```python
from build123d import *

# Parameters (mm, degrees)
SKETCH1_W                = 23.7998
SKETCH1_H                = 9.525
BOSS_EXTRUDE1_DEPTH      = 4.7625
BOSS_EXTRUDE1_DEPTH_BACK = 4.7625
SKETCH2_W                = 14.2748
SKETCH2_H                = 5.08
CUT_EXTRUDE1_DEPTH       = 4.7625
CUT_EXTRUDE1_DEPTH_BACK  = 4.7625
HOLE1_D                  = 3.96748
HOLE1_DEPTH              = 7.874
HOLE1_CSINK_D            = 4.826
HOLE1_CSINK_ANGLE        = 90
HOLE2_D                  = 3.96748
HOLE2_DEPTH              = 1.651
HOLE3_D                  = 4.826
HOLE3_DEPTH              = 9.525


with BuildPart() as part:
    # Sketch1 → Boss-Extrude1 (new body, two sides)
    with BuildSketch(Plane.XY) as boss_extrude1_sk:
        with Locations((7.1501, 0)):
            Rectangle(SKETCH1_W, SKETCH1_H)
    extrude(amount=BOSS_EXTRUDE1_DEPTH)
    extrude(boss_extrude1_sk.sketch, amount=-BOSS_EXTRUDE1_DEPTH_BACK)

    # Sketch2 → Cut-Extrude1 (cut, two sides)
    with BuildSketch(Plane(origin=(0, 0, 0), x_dir=(1, 0, 0), z_dir=(0, 1, 0))) as cut_extrude1_sk:
        with Locations((2.3876, 0)):
            Rectangle(SKETCH2_W, SKETCH2_H)
    extrude(amount=CUT_EXTRUDE1_DEPTH, mode=Mode.SUBTRACT)
    extrude(cut_extrude1_sk.sketch, amount=-CUT_EXTRUDE1_DEPTH_BACK, mode=Mode.SUBTRACT)

    # Hole1
    with Locations(Plane(origin=(19.05, 0, 0), x_dir=(0, 0, -1), z_dir=(1, 0, 0))):
        with Locations((0, 0)):
            CounterSinkHole(HOLE1_D / 2, HOLE1_CSINK_D / 2, depth=HOLE1_DEPTH, counter_sink_angle=HOLE1_CSINK_ANGLE)

    # Hole2
    with Locations(Plane(origin=(11.176, 0, 0), x_dir=(0, 0, -1), z_dir=(1, 0, 0))):
        with Locations((0, 0)):
            Hole(HOLE2_D / 2, depth=HOLE2_DEPTH)

    # Hole3
    with Locations(Plane(origin=(0, 0, -4.7625), x_dir=(-1, 0, 0), z_dir=(0, 0, -1))):
        with Locations((0, 0)):
            Hole(HOLE3_D / 2, depth=HOLE3_DEPTH)

    # Sketch9 → Cut-Revolve1 (revolve, cut)
    with BuildSketch(Plane.XY):
        with BuildLine():
            Line((19.05, 0), (19.05, 4.7625))
            ThreePointArc((19.05, 4.7625), (18.092047749, 7.310175466), (16.51, 9.525))
            Line((16.51, 9.525), (23.8125, 9.525))
            Line((23.8125, 9.525), (23.8125, 0))
            Line((23.8125, 0), (19.05, 0))
        make_face()
    revolve(axis=Axis((23.8125, 0, 0), (-1, 0, 0)), mode=Mode.SUBTRACT)

    # Sketch10 → Cut-Revolve2 (revolve, cut)
    with BuildSketch(Plane.XY):
        with BuildLine():
            Line((-9.5123, 0), (-9.5123, 9.525))
            Line((-9.5123, 9.525), (-2.2098, 9.525))
            ThreePointArc((-2.2098, 9.525), (-3.791847749, 7.310175466), (-4.7498, 4.7625))
            Line((-4.7498, 4.7625), (-4.7498, 0))
            Line((-4.7498, 0), (-9.5123, 0))
        make_face()
    revolve(axis=Axis((-4.7498, 0, 0), (-1, 0, 0)), mode=Mode.SUBTRACT)


solid = part.part
```
Geometry: final body of the model. Coordinates: model frame, mm. A direction names the side the tool comes from. Coordinates: 2 decimals unless noted, no trailing zeros. Order: outer loops, then holes, each group sorted by start corner. A loop starts at its lowest first (then second) coordinate and runs counter-clockwise, first axis right, second up. Notation, with made-up numbers: (84, 57.25) - (124, 57.25) arc R13 ccw to (124, 70.25) - close; hole circle Ø3 at (-25.5, -0.5). An arc over 180 degrees is marked (long way). Return JSON: item names as keys, results as strings. Group by question number.
1. Pull-direction query (Y, two-part tool) for faces 3 (the face through (-1.915, -1.468, 3.667)), 4 (the face through (10, -4.762, 0)), 5 (the face through (4, 0, 2.54)); classes: pulls with the +Y half, pulls with the -Y half, needs draft (parallel to the pull), parting line crosses it, or undercut.
2. Pin query (flat end, axial travel): pin 1 (4.5 mm diameter, centred on y = 0, z = 0, fed in from -X) (3 decimals); pin 2 (4.5 mm diameter, centred on x = 0, y = 0, fed in from -Z). Return the tip coordinate at first contact, or that it passes through.
3. Set-up query: faces 1 (the face through (-4.75, 0, 3)), 2 (the face through (9.525, 1, 2)). Return all of +Z, -Z, +X, -X, +Y, -Y with unobstructed straight access to the full face (end or side cutting, diameter ignored); none if empty.
4. Material intervals for line 1 along Y through (x, z) = (0, -4.1); line 2 along Z through (x, y) = (7.25, -2); line 3 along Z through (x, y) = (15.5, 1.25), sorted ascending. Write a range as [from, to].
5. Cut plane C-C (x = 13.75). Output: boundary loops of the cut face in (y, z), plus the area to 3 significant figures.
6. Cut plane B-B (x = -3). Output: boundary loops of the cut face in (y, z).
7. Cut plane A-A (x = 0). Output: boundary loops of the cut face in (y, z), plus the area to 3 significant figures.
Resolved:
{
 "1": {"face 3": "undercut", "face 4": "pulls with the -Y half", "face 5": "needs draft"},
 "2": {"pin 1": "stops at x = 9.525", "pin 2": "passes through"},
 "3": {"face 1": "+Z, -Z, -X, +Y, -Y", "face 2": "-X, +Y, -Y"},
 "4": {"line 1": "y = [-4.76, -2.41], [2.41, 4.76]", "line 2": "z = [-4.76, -2.54], [2.54, 4.76]", "line 3": "z = [-4.76, -1.54], [1.54, 4.76]"},
 "5": {"outline": "(-4.76, -4.76) - (4.76, -4.76) - (4.76, 4.76) - (-4.76, 4.76) - close; hole circle Ø3.97 at (0, 0)", "area": "78.4 mm²"},
 "6": {"outline": "(-4.76, -4.76) - (4.76, -4.76) - (4.76, -2.54) - (-4.76, -2.54) - close; (-4.76, 2.54) - (4.76, 2.54) - (4.76, 4.76) - (-4.76, 4.76) - close"},
 "7": {"outline": "(-4.76, -4.76) - (-2.41, -4.76) - (-2.41, -2.54) - (-4.76, -2.54) - close; (-4.76, 2.54) - (-2.41, 2.54) - (-2.41, 4.76) - (-4.76, 4.76) - close; (2.41, -4.76) - (4.76, -4.76) - (4.76, -2.54) - (2.41, -2.54) - close; (2.41, 2.54) - (4.76, 2.54) - (4.76, 4.76) - (2.41, 4.76) - close", "area": "20.9 mm²"}
}
